from build123d import *

# Parameters (mm, degrees)
SKETCH1_W           = 160
SKETCH1_H           = 66
BOSS_EXTRUDE1_DEPTH = 40
SKETCH2_R           = 4.025
SKETCH2_W           = 130
SKETCH2_H           = 37.5
CUT_EXTRUDE1_DEPTH  = 112.157545853
SKETCH3_R           = 1
SKETCH3_W           = 120
SKETCH3_H           = 20
CUT_EXTRUDE2_DEPTH  = 96.336247042
SKETCH4_R           = 12.5
CUT_EXTRUDE3_DEPTH  = 95.314633011


with BuildPart() as part:
    # Sketch1 → Boss-Extrude1 (new body)
    with BuildSketch(Plane(origin=(0, 0, 0), x_dir=(1, 0, 0), z_dir=(0, 1, 0))):
        Rectangle(SKETCH1_W, SKETCH1_H)
    extrude(amount=BOSS_EXTRUDE1_DEPTH)

    # Sketch2 → Cut-Extrude1 (cut, through all)
    with BuildSketch(Plane.XY.offset(33)):
        with Locations((70, 20)):
            Circle(SKETCH2_R)
        with Locations((-15, 21.25)):
            Rectangle(SKETCH2_W, SKETCH2_H)
    extrude(amount=-CUT_EXTRUDE1_DEPTH, mode=Mode.SUBTRACT)

    # Sketch3 → Cut-Extrude2 (cut, through all)
    with BuildSketch(Plane(origin=(0, 40, 0), x_dir=(1, 0, 0), z_dir=(0, 1, 0))):
        with Locations(Location((-75, 30, 0), (0, 0, 270))):
            Circle(SKETCH3_R)
        with Locations(Location((-75, 3, 0), (0, 0, 270))):
            Circle(SKETCH3_R)
        with Locations(Location((-67, 30, 0), (0, 0, 270))):
            Circle(SKETCH3_R)
        with Locations(Location((-59, 30, 0), (0, 0, 270))):
            Circle(SKETCH3_R)
        with Locations(Location((-51, 30, 0), (0, 0, 270))):
            Circle(SKETCH3_R)
        with Locations(Location((-67, 3, 0), (0, 0, 270))):
            Circle(SKETCH3_R)
        with Locations(Location((-59, 3, 0), (0, 0, 270))):
            Circle(SKETCH3_R)
        with Locations(Location((-51, 3, 0), (0, 0, 270))):
            Circle(SKETCH3_R)
        with Locations(Location((-6.5, 30, 0), (0, 0, 270))):
            Circle(SKETCH3_R)
        with Locations(Location((-6.5, 3, 0), (0, 0, 270))):
            Circle(SKETCH3_R)
        with Locations(Location((1.5, 30, 0), (0, 0, 270))):
            Circle(SKETCH3_R)
        with Locations(Location((9.5, 30, 0), (0, 0, 270))):
            Circle(SKETCH3_R)
        with Locations(Location((17.5, 30, 0), (0, 0, 270))):
            Circle(SKETCH3_R)
        with Locations(Location((1.5, 3, 0), (0, 0, 270))):
            Circle(SKETCH3_R)
        with Locations(Location((9.5, 3, 0), (0, 0, 270))):
            Circle(SKETCH3_R)
        with Locations(Location((17.5, 3, 0), (0, 0, 270))):
            Circle(SKETCH3_R)
        with Locations((17.5, -3)):
            Circle(SKETCH3_R)
        with Locations((9.5, -3)):
            Circle(SKETCH3_R)
        with Locations((1.5, -3)):
            Circle(SKETCH3_R)
        with Locations((17.5, -30)):
            Circle(SKETCH3_R)
        with Locations((9.5, -30)):
            Circle(SKETCH3_R)
        with Locations((1.5, -30)):
            Circle(SKETCH3_R)
        with Locations((-6.5, -3)):
            Circle(SKETCH3_R)
        with Locations((-6.5, -30)):
            Circle(SKETCH3_R)
        with Locations((-51, -3)):
            Circle(SKETCH3_R)
        with Locations((-59, -3)):
            Circle(SKETCH3_R)
        with Locations((-67, -3)):
            Circle(SKETCH3_R)
        with Locations((-51, -30)):
            Circle(SKETCH3_R)
        with Locations((-59, -30)):
            Circle(SKETCH3_R)
        with Locations((-67, -30)):
            Circle(SKETCH3_R)
        with Locations((-75, -3)):
            Circle(SKETCH3_R)
        with Locations((-75, -30)):
            Circle(SKETCH3_R)
        with Locations((-17.5, 16.5)):
            Rectangle(SKETCH3_W, SKETCH3_H)
        with Locations((-17.5, -16.5)):
            Rectangle(SKETCH3_W, SKETCH3_H)
    extrude(amount=-CUT_EXTRUDE2_DEPTH, mode=Mode.SUBTRACT)

    # Sketch4 → Cut-Extrude3 (cut, through all)
    with BuildSketch(Plane(origin=(0, 2.5, 0), x_dir=(1, 0, 0), z_dir=(0, 1, 0))):
        with Locations((-44.25, -16.5)):
            Circle(SKETCH4_R)
        with Locations((-44.25, 16.5)):
            Circle(SKETCH4_R)
        with Locations((-13.25, 16.5)):
            Circle(SKETCH4_R)
        with Locations((-13.25, -16.5)):
            Circle(SKETCH4_R)
    extrude(amount=-CUT_EXTRUDE3_DEPTH, mode=Mode.SUBTRACT)


solid = part.part
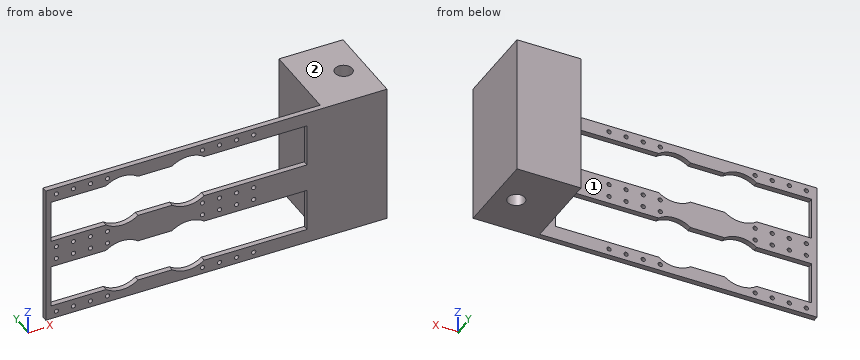
Verification items for the finished model (mm, model axes). Face numbers are marked on the shaded views. A direction names the side the tool comes from. Round coordinates to 2 decimals unless told otherwise and drop trailing zeros. Loops run counter-clockwise (first coordinate to the right, second up) from the corner with the lowest first, then second, coordinate; pieces in that order, holes last. Notation, with made-up numbers: (12.25, 76) - (59.25, 76) arc R30 cw to (59.25, 109) - close; hole circle Ø1 at (32.25, -14.75). An arc over 180 degrees is marked (long way). Answer in a Markdown table with one row per item. Add a question column.
Q1. Section check A-A on z = 20.5. Enter the section's corners in (x, y) (3 decimals), plus the area to 3 significant figures.
Q2. Section check B-B on x = 70. Enter the section's corners in (y, z) (3 decimals), plus the area to 3 significant figures.
Q3. Material ranges on line 1 (X direction, y = 30, z = 24.5); line 2 (Y direction, x = 32.5, z = 6); line 3 (X direction, y = 22, z = 6), recorded low to high.
Q4. Section check C-C on y = 20. Enter the section's corners in (x, z) (3 decimals).
Q5. Section check D-D on x = 34.5. Enter the section's corners in (y, z).
Q6. Tool access check on the marked faces 1 and 2. Record the directions out of +Z, -Z, +X, -X, +Y, -Y that give a thin tool (end or side, any length) a straight path to the whole face; none if there is none.
Q7. Gauge pin test, flat ends, axial feed: pin 1 (1.5 mm diameter, centred on y = 34.5, z = 16.5, fed in from -X); pin 2 (2.5 mm diameter, centred on x = -6.5, z = 3, fed in from +Y). Record the tip position at first contact, or that the pin passes through.
Found:
| question | item | result |
|---|---|---|
| 1 | outline | (-80, 0) - (-77.5, 0) - (-77.5, 2.5) - (-80, 2.5) - close; (42.5, 0) - (80, 0) - (80, 40) - (50, 40) - (50, 2.5) - (42.5, 2.5) - close; hole circle Ø8.05 at (70, 20) |
| 1 | area | 1,170 mm² |
| 2 | outline | (0, -33) - (15.975, -33) - (15.975, 33) - (0, 33) - close; (24.025, -33) - (40, -33) - (40, 33) - (24.025, 33) - close |
| 2 | area | 2,110 mm² |
| 3 | line 1 | x = 50 to 80 |
| 3 | line 2 | y = 0 to 2.5 |
| 3 | line 3 | x = 50 to 66.51, 73.49 to 80 |
| 4 | outline | (50, -33) - (65.975, -33) - (65.975, 33) - (50, 33) - close; (74.025, -33) - (80, -33) - (80, 33) - (74.025, 33) - close |
| 5 | outline | (0, -33) - (2.5, -33) - (2.5, -26.5) - (0, -26.5) - close; (0, -6.5) - (2.5, -6.5) - (2.5, 6.5) - (0, 6.5) - close; (0, 26.5) - (2.5, 26.5) - (2.5, 33) - (0, 33) - close |
| 6 | face 1 | +Z, -Z, -X, +Y |
| 6 | face 2 | +Z, +X, -X, +Y, -Y |
| 7 | pin 1 | stops at x = 50 |
| 7 | pin 2 | stops at y = 2.5 |
